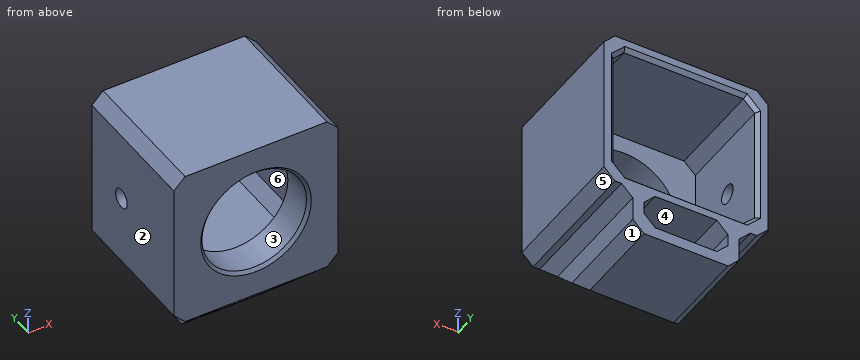
```python
from build123d import *

# Parameters (mm, degrees)
F0_W        = 44
F0_H        = 43
F0_W_2      = 38
F0_H_2      = 37
F1_DEPTH    = 27.2
F2_W        = 44
F2_H        = 43
F2_R        = 14
F3_DEPTH    = 9
F4_SIZE     = 3
F6_DEPTH    = 36.2
F7_SIZE     = 3
F8_T1_DEPTH = 85.763401504
F9_R        = 2.55
F10_DEPTH   = 3
F11_SIZE    = 0.8
F12_SIZE    = 1


# Not quite as in the source:
# - a fillet or chamfer that OpenCascade refuses, or shapes differently, is made with other operations: its cross-section is extruded or revolved along the edge and cut away or added


with BuildPart() as f1:
    # F0 (on Front) → F1 (new body)
    with BuildSketch(Plane.XZ):
        Rectangle(F0_W, F0_H)
        Rectangle(F0_W_2, F0_H_2, mode=Mode.SUBTRACT)
    extrude(amount=F1_DEPTH)

    # F2 (on face) → F3 (join)
    with BuildSketch(Plane.XZ.offset(27.2)):
        Rectangle(F2_W, F2_H)
        Circle(F2_R, mode=Mode.SUBTRACT)
    extrude(amount=F3_DEPTH)

    # F4
    f4_edges = [f1.edges().sort_by_distance(p)[0] for p in [
        (22, -18.1, 21.5),
        (22, -18.1, -21.5),
        (-22, -18.1, -21.5),
        (-22, -18.1, 21.5),
        (-19, -13.6, 18.5),
        (-19, -13.6, -18.5),
        (19, -13.6, -18.5),
        (19, -13.6, 18.5),
    ]]
    chamfer(f4_edges, length=F4_SIZE)

    # F5 (on face) → F6 (join, through all)
    with BuildSketch(Plane.XZ.offset(36.2)):
        Polygon((-14.25, -33.8), (14.25, -33.8), (14.25, -21.5), (11.25, -21.5), (11.25, -30.8), (-11.25, -30.8), (-11.25, -21.5), (-14.25, -21.5), align=None)
    extrude(amount=-F6_DEPTH)

    # F7
    f7_edges = [f1.edges().sort_by_distance(p)[0] for p in [
        (-14.25, -18.1, -33.8),
        (-14.25, -18.1, -21.5),
        (-11.25, -18.1, -30.8),
        (11.25, -18.1, -30.8),
        (11.25, -18.1, -21.5),
        (14.25, -18.1, -33.8),
        (14.25, -18.1, -21.5),
        (-11.25, -18.1, -21.5),
    ]]
    chamfer(f7_edges, length=F7_SIZE)

    # F8: chamfer of 12.3 on 1 edges, made by hand

    # F8_s2 → F8_t1 (cut)
    with BuildSketch(Plane.YZ.offset(-42.881700752)):
        Polygon((-36.2, -21.5), (-23.9, -33.8), (-36.2, -33.8), align=None)
    extrude(amount=F8_T1_DEPTH, mode=Mode.SUBTRACT)

    # F9 (on face) → F10 (cut, through all)
    with BuildSketch(Plane(origin=(-22, 0, 0), x_dir=(0, -1, 0), z_dir=(-1, 0, 0))):
        with Locations((13.05, 0)):
            Circle(F9_R)
    extrude(amount=-F10_DEPTH, mode=Mode.SUBTRACT)

    # F11
    f11_edges = [f1.edges().sort_by_distance(p)[0] for p in [
        (-14, -36.2, 0),
    ]]
    chamfer(f11_edges, length=F11_SIZE)

    # F12
    f12_edges = [f1.edges().sort_by_distance(p)[0] for p in [
        (0, 0, 18.5),
        (19, 0, 0),
        (0, 0, -18.5),
        (-19, 0, 0),
        (17.5, 0, 17),
        (17.5, 0, -17),
        (-17.5, 0, -17),
        (-17.5, 0, 17),
    ]]
    chamfer(f12_edges, length=F12_SIZE)


solid = f1.part
```
Check sheet for the modelled part. Datum: model origin and axes. Units: mm. Face numbers are marked on the shaded views. A direction names the side the tool comes from. Give positions to 0.01 mm unless a question says otherwise; leave off trailing zeros. Order: outer loops, then holes, each group sorted by start corner. A loop starts at its lowest first (then second) coordinate and runs counter-clockwise, first axis right, second up. Notation, with made-up numbers: (83, -13) -> (97, -13) arc R29 ccw to (97, 23) -> close; hole circle Ø2 at (4, 70.25). An arc over 180 degrees is marked (long way). Return JSON: item names as keys, results as strings.
1. Material ranges on probe 1 along Z at (x, y) = (0, -31); probe 2 along Z at (x, y) = (1, -27); probe 3 along X at (y, z) = (-3, 14), recorded low to high. Write a range as [from, to].
From the geometry:
{"probe 1": "[-21.5, -14], [14, 21.5]", "probe 2": "[-21.5, -18.5], [18.5, 21.5]", "probe 3": "[-22, -19], [19, 22]"}
2. Cross-section at B-B, the plane y = -17. Count the separate pieces of the cut face and the enclosed holes in it, plus the area to 3 significant figures.
From the geometry:
{"separate pieces": "1", "enclosed holes": "2", "area": "645 mm^2"}
3. Cross-section at D-D, the plane y = -32. Record the cut outline in (x, z).
From the geometry:
{"outline": "(-22, -18.5) -> (-19, -21.5) -> (-17.25, -21.5) -> (-14.25, -24.5) -> (-14.25, -25.7) -> (-11.25, -25.7) -> (-11.25, -24.5) -> (-8.25, -21.5) -> (8.25, -21.5) -> (11.25, -24.5) -> (11.25, -25.7) -> (14.25, -25.7) -> (14.25, -24.5) -> (17.25, -21.5) -> (19, -21.5) -> (22, -18.5) -> (22, 18.5) -> (19, 21.5) -> (-19, 21.5) -> (-22, 18.5) -> close; hole circle Ø28 at (0, 0)"}
4. Cross-section at A-A, the plane z = 0. Record the cut outline in (x, y), plus the area to 3 significant figures.
From the geometry:
{"outline": "(-22, -36.2) -> (-14.8, -36.2) -> (-14, -35.4) -> (-14, -27.2) -> (-19, -27.2) -> (-19, -15.6) -> (-22, -15.6) -> close; (-22, -10.5) -> (-19, -10.5) -> (-19, -1) -> (-20, 0) -> (-22, 0) -> close; (14, -35.4) -> (14.8, -36.2) -> (22, -36.2) -> (22, 0) -> (20, 0) -> (19, -1) -> (19, -27.2) -> (14, -27.2) -> close", "area": "290 mm^2"}
5. Mould release check, pull along X, two halves, no side actions. Record for the marked faces 1, 2 and 3: +X half, -X half, draft (parallel to the pull), parting line (faces both ways), or undercut.
From the geometry:
{"face 1": "+X half", "face 2": "-X half", "face 3": "undercut"}
6. Cross-section at C-C, the plane x = 0. Record the cut outline in (y, z), plus the area to 3 significant figures.
From the geometry:
{"outline": "(-36.2, -21.5) -> (0, -21.5) -> (0, -19.5) -> (-1, -18.5) -> (-27.2, -18.5) -> (-27.2, -14) -> (-35.4, -14) -> (-36.2, -14.8) -> close; (-36.2, 14.8) -> (-35.4, 14) -> (-27.2, 14) -> (-27.2, 18.5) -> (-1, 18.5) -> (0, 19.5) -> (0, 21.5) -> (-36.2, 21.5) -> close; (-26.9, -30.8) -> (-23.9, -33.8) -> (0, -33.8) -> (0, -30.8) -> close", "area": "373 mm^2"}
7. Set-up check for the marked faces 4, 5 and 6: record each of +Z, -Z, +X, -X, +Y, -Y from which the full face is reachable in a straight line by a thin tool's end or side.
From the geometry:
{"face 4": "+Y, -Y", "face 5": "-Z, +X, +Y, -Y", "face 6": "+Y"}
8. Go/stop test with flat-tipped pins: P1, Ø3.5, axis at y = -24, z = -27, coming from the -X side; P2, Ø1.9, axis at x = -17.5, y = -22, coming from the -Z side; P3, Ø2.5, axis at y = -19, z = -26.5, coming from the +X side. Record where each tip stops, or that it passes through.
From the geometry:
{"P1": "x = -14.25", "P2": "z = -22.2", "P3": "x = 14.25"}
